Read the model definition and answer for the solid it produces. Units are mm, in the model's axes. A direction names the side the tool comes from. Coordinates: 2 decimals unless noted, no trailing zeros. Order: outer loops, then holes, each group sorted by start corner. A loop starts at its lowest first (then second) coordinate and runs counter-clockwise, first axis right, second up. Notation, with made-up numbers: (74.5, -33.75) -> (90.5, -33.75) arc R15 ccw to (90.5, -6.75) -> close; hole circle Ø2 at (22.5, 82). An arc over 180 degrees is marked (long way). Answer in a Markdown table with one row per item.
Autodesk Inventor part; units mm, degrees
ref_plane "YZ Plane" through (0, 0, 0) normal (1, 0, 0) x (0, 1, 0)
ref_plane "XZ Plane" through (0, 0, 0) normal (0, 1, 0) x (-1, 0, 0)
ref_plane "XY Plane" through (0, 0, 0) normal (0, 0, 1) x (1, 0, 0)
sketch "草图1" plane through (0, 0, 0) normal (0, 1, 0) x (-1, 0, 0)
  point P0 (0, 0)
sketch "草图2" plane through (0, 0, 0) normal (0, 1, 0) x (-1, 0, 0)
  line L0 (0, 0) -> (-2.5, 0)
  line L1 (-2.5, 0) -> (-2.5, -5.3)
  line L2 (-2.5, -5.3) -> (0, -5.3)
  line L3 (0, -5.3) -> (0, 0)
  dimension "d0" = 2.5
  dimension "d1" = 5.3
extrude "拉伸1" add sketch "草图2" along normal blind 1.5
sketch "草图3" plane through (0, 1.5, 0) normal (0, 1, 0) x (1, 0, 0)
  line L0 (2.5, 5.3) -> (0, 5.3)
  line L1 (1.25, 5.3) -> (1.25, 0)
  line L2 (0, 5.3) -> (0, 0)
  line L3 (1.25, 2.65) -> (1.25, 3.92)
  line L4 (1.25, 3.92) -> (1.25, 1.38)
  circle A0 centre (1.25, 3.92) radius 1
  circle A1 centre (1.25, 1.38) radius 1
  dimension "d4" = 1.27
  dimension "d5" = 2.54
  dimension "d6" = 2
  dimension "d7" = 2
extrude "拉伸2" add sketch "草图3" along normal blind 0.5
sketch "草图4" plane through (1.25, 2, -1.38) normal (0, 1, 0) x (1, 0, 0)
  circle A0 centre (0, 0) radius 0.4
  circle A1 centre (0, 2.54) radius 1
  circle A2 centre (0, 2.54) radius 0.4
  point P0 (-1.25, -1.38)
  dimension "d10" = 0.8
  dimension "d11" = 0.8
extrude "拉伸3" add sketch "草图4" along normal blind 2 contours A0 | A2
sketch "草图5" plane through (0, 0, 0) normal (0, -1, 0) x (1, 0, 0)
  circle A0 centre (1.25, -3.92) radius 0.4
  circle A1 centre (1.25, -3.92) radius 0.725
  circle A2 centre (1.25, -1.38) radius 0.4
  circle A3 centre (1.25, -1.38) radius 0.725
  point P0 (0, 0)
  dimension "d14" = 1.45
  dimension "d15" = 1.45
extrude "拉伸4" add sketch "草图5" along normal blind 4 contours A0 | A1 | A2 | A3
sketch "草图6" plane through (1.25, -4, -1.38) normal (0, -1, 0) x (1, 0, 0)
  circle A0 centre (0, 0) radius 0.45
  circle A1 centre (0, -2.54) radius 0.725
  circle A2 centre (0, -2.54) radius 0.45
  point P0 (-1.25, 1.38)
  dimension "d18" = 0.9
  dimension "d19" = 0.9
extrude "拉伸5" add sketch "草图6" along normal blind 2 contours A0 | A2
fillet "圆角1" radius 0.45 1 edges at (0.8, -6, -3.92)
fillet "圆角2" radius 0.45 1 edges at (0.8, -6, -1.38)
fillet "圆角3" radius 0.15 2 edges at (0.525, -4, -3.92) (0.525, -4, -1.38)
properties part number "Pogo_Pin" material "铜"
Q1. The part is cut by section B-B (y = -2.75). Write down the section's boundary in (x, z) (3 decimals).
Outcome:
| item | result |
|---|---|
| outline | circle Ø1.45 at (1.25, -3.92); circle Ø1.45 at (1.25, -1.38) |
Q2. Given pin 1 (1 mm diameter, centred on x = 1.5, z = -3.5, fed in from +Y); pin 2 (1.2 mm diameter, centred on x = 0.5, z = -3, fed in from +Y), each flat-ended and moving along its own axis, determine where each tip first touches the part or whether it passes through.
Outcome:
| item | result |
|---|---|
| pin 1 | y = 4 |
| pin 2 | y = 2 |
Q3. The part is cut by section A-A (z = -3.92). Write down the section's boundary in (x, y) (3 decimals), then the cut area to 3 significant figures.
Outcome:
| item | result |
|---|---|
| outline | (0, 0) -> (0.525, 0) -> (0.525, -3.85) arc R0.15 ccw to (0.675, -4) -> (0.8, -4) -> (0.8, -5.55) arc R0.45 ccw to (1.7, -5.55) -> (1.7, -4) -> (1.825, -4) arc R0.15 ccw to (1.975, -3.85) -> (1.975, 0) -> (2.5, 0) -> (2.5, 1.5) -> (2.25, 1.5) -> (2.25, 2) -> (1.65, 2) -> (1.65, 4) -> (0.85, 4) -> (0.85, 2) -> (0.25, 2) -> (0.25, 1.5) -> (0, 1.5) -> close |
| area | 13.9 mm² |
Q4. Consider line 1 (Z direction, x = 1.3, y = -5.25); line 2 (Y direction, x = 2, z = -1.85); line 3 (Z direction, x = 0.45, y = 1.75). Determine where each line is inside the solid, lowest interval first.
Outcome:
| item | result |
|---|---|
| line 1 | -4.37 to -3.47, -1.83 to -0.93 |
| line 2 | 0 to 2 |
| line 3 | -4.52 to -3.32, -1.98 to -0.78 |
Q5. For faces 1 (the face through (1, 0, -3)), 2 (the face through (0, 1, -3)), 3 (the face through (1.3, 1.5, -2.6)), determine the directions among +Z, -Z, +X, -X, +Y, -Y from which every point of the face is accessible in a straight line to the end or side of a thin tool.
Outcome:
| item | result |
|---|---|
| face 1 | -Y |
| face 2 | +Z, -Z, -X, +Y, -Y |
| face 3 | +Y |
Q6. For a pull along Z with two mould halves and no side action, classify faces 4 (the face through (1.666, -4.764, -1.208)), 5 (the face through (2.5, 1, -3)), 6 (the face through (1, 1, -5.3)) as pulls with the +Z half, pulls with the -Z half, needs draft (parallel to the pull), parting line crosses it, or undercut.
Outcome:
| item | result |
|---|---|
| face 4 | undercut |
| face 5 | needs draft |
| face 6 | pulls with the -Z half |
